```python
from build123d import *

# Parameters (mm, degrees)
BOSS_EXTRUDE1_DEPTH        = 25.4
F_10_32_TAPPED_HOLE1_D     = 4.0386
F_10_32_TAPPED_HOLE1_DEPTH = 13.716
F_10_32_TAPPED_HOLE1_TIP   = 1.213317848
F_9_0_196_DIAMETER_HOLE1_D = 4.9784


with BuildPart() as part:
    # Sketch1 → Boss-Extrude1 (new body)
    with BuildSketch(Plane(origin=(0, 0, 0), x_dir=(0, 0, -1), z_dir=(1, 0, 0))):
        Polygon((82.55, 0), (79.375, 0), (79.375, 34.925), (3.175, 34.925), (3.175, 0), (0, 0), (0, 38.1), (82.55, 38.1), align=None)
    extrude(amount=BOSS_EXTRUDE1_DEPTH)

    # #10-32 Tapped Hole1
    with Locations(Plane(origin=(0, 38.1, 0), x_dir=(1, 0, 0), z_dir=(0, 1, 0))):
        with Locations((16.764, 41.275)):
            Hole(F_10_32_TAPPED_HOLE1_D / 2, depth=F_10_32_TAPPED_HOLE1_DEPTH)
            with Locations((0, 0, -(F_10_32_TAPPED_HOLE1_DEPTH + F_10_32_TAPPED_HOLE1_TIP / 2))):  # 118° drill point
                Cone(0, F_10_32_TAPPED_HOLE1_D / 2, F_10_32_TAPPED_HOLE1_TIP, mode=Mode.SUBTRACT)

    # #9 (0.196) Diameter Hole1 (through all)
    with Locations(Plane.XY):
        with Locations((6.35, 6.35), (19.05, 6.35)):
            Hole(F_9_0_196_DIAMETER_HOLE1_D / 2)


solid = part.part
```
Model file for the job. Use its own axes, mm. A direction names the side the tool comes from. Give positions to 0.01 mm unless a question says otherwise; leave off trailing zeros. Loops run counter-clockwise (first coordinate to the right, second up) from the corner with the lowest first, then second, coordinate; pieces in that order, holes last. Notation, with made-up numbers: M 58,61.5 L 74,61.5 A20 ccw 74,94.5 Z; hole C 40.25,-3 d2. An arc over 180 degrees is marked long. Use one line per item in the form item = value.
Item 1: Slice it at A-A on y = 6.35. List the corners of the cut face in (x, z) (3 decimals), and give its area (3 significant figures).
Filled in:
outline = M 0,-82.55 L 3.861,-82.55 L 3.861,-79.375 L 0,-79.375 Z; M 0,-3.175 L 3.861,-3.175 L 3.861,0 L 0,0 Z; M 8.839,-82.55 L 16.561,-82.55 L 16.561,-79.375 L 8.839,-79.375 Z; M 8.839,-3.175 L 16.561,-3.175 L 16.561,0 L 8.839,0 Z; M 21.539,-82.55 L 25.4,-82.55 L 25.4,-79.375 L 21.539,-79.375 Z; M 21.539,-3.175 L 25.4,-3.175 L 25.4,0 L 21.539,0 Z
area = 98.1 mm^2
Item 2: Two-plate mould, pull along Z, no slides. Class faces 1 (the cylindrical face through (5.201, 4.142, -1.61)), 2 (the flat face through (13, 19, 0)), 3 (the flat face through (13, 34.925, -42)): released by +Z, released by -Z, zero draft, split by the parting line, or undercut.
Filled in:
face_1 = zero draft
face_2 = released by +Z
face_3 = undercut
Item 3: Which spindle directions (+Z, -Z, +X, -X, +Y, -Y) get a long thin tool onto all of the face, cutting with end or side? Do faces 4 (the flat face through (13, 17, -79.375)), 5 (the flat face through (13, 19, -82.55)). Say none if no direction does.
Filled in:
face_4 = +X, -X, -Y
face_5 = -Z, +X, -X, +Y, -Y
Item 4: Flat gauge pins, fed straight in: pin 1 Ø3 at (x, z) = (11, -67.5) entering from -Y (3 decimals); pin 2 Ø4.5 at (x, y) = (6.35, 6.35) entering from -Z. Where does each tip first touch, or does it go through?
Filled in:
pin_1 = 34.925
pin_2 = through
Item 5: Slice it at C-C on y = 19. List the corners of the cut face in (x, z) (3 decimals).
Filled in:
outline = M 0,-82.55 L 25.4,-82.55 L 25.4,-79.375 L 0,-79.375 Z; M 0,-3.175 L 25.4,-3.175 L 25.4,0 L 0,0 Z
Item 6: Drill centre lines: L1, parallel to Z at x = 8, y = 2.5 (3 decimals); L2, parallel to X at y = 6, z = -80. Where is each one in solid material? Low to high.
Filled in:
L1 = -82.55 to -79.375, -3.175 to 0
L2 = 0 to 3.89, 8.81 to 16.59, 21.51 to 25.4
Item 7: Slice it at B-B on x = 6.35. List the corners of the cut face in (y, z) (3 decimals), and give its area (3 significant figures).
Filled in:
outline = M 0,-82.55 L 3.861,-82.55 L 3.861,-79.375 L 0,-79.375 Z; M 0,-3.175 L 3.861,-3.175 L 3.861,0 L 0,0 Z; M 8.839,-82.55 L 38.1,-82.55 L 38.1,0 L 8.839,0 L 8.839,-3.175 L 34.925,-3.175 L 34.925,-79.375 L 8.839,-79.375 Z
area = 452 mm^2
Item 8: Slice it at D-D on x = 23.75. List the corners of the cut face in (y, z) (3 decimals), and give its area (3 significant figures).
Filled in:
outline = M 0,-82.55 L 38.1,-82.55 L 38.1,0 L 0,0 L 0,-3.175 L 34.925,-3.175 L 34.925,-79.375 L 0,-79.375 Z
area = 484 mm^2
